Verification items for the finished model (mm, model axes). A direction names the side the tool comes from. Give positions to 0.01 mm unless a question says otherwise; leave off trailing zeros. Write each loop counter-clockwise with the first axis right and the second up, starting at its lowest first coordinate (ties: lowest second). Pieces come first, ordered by that corner, then holes. Notation, with made-up numbers: (-28.5, 42.5) -> (-19.5, 42.5) arc R22 cw to (-19.5, 76.5) -> close; hole circle Ø11 at (25.25, 76.25). An arc over 180 degrees is marked (long way). Answer as CSV lines item,"result".
```python
from build123d import *

# Parameters (mm, degrees)
F0_W     = 120
F0_H     = 118
F1_DEPTH = 4
F2_W     = 1
F2_H     = 1
F2_W_2   = 113
F2_H_2   = 111
F3_DEPTH = 2.5
F4_W     = 113
F4_H     = 111
F5_DEPTH = 5
F6_R     = 4


with BuildPart() as f1:
    # F0 (on Top) → F1 (new body)
    with BuildSketch(Plane.XY):
        Rectangle(F0_W, F0_H)
    extrude(amount=F1_DEPTH)

    # F2 (on face) → F3 (join)
    with BuildSketch(Plane.XY.offset(4)):
        with Locations((-57, 56)):
            Rectangle(F2_W, F2_H)
        with Locations((0, 56)):
            Rectangle(F2_W_2, F2_H)
        with Locations((-57, 0)):
            Rectangle(F2_W, F2_H_2)
        with Locations((57, 56)):
            Rectangle(F2_W, F2_H)
        with Locations((-57, -56)):
            Rectangle(F2_W, F2_H)
        with Locations((0, -56)):
            Rectangle(F2_W_2, F2_H)
        with Locations((57, 0)):
            Rectangle(F2_W, F2_H_2)
        with Locations((57, -56)):
            Rectangle(F2_W, F2_H)
    extrude(amount=F3_DEPTH)

    # F4 (on face) → F5 (cut)
    with BuildSketch(Plane.XY.offset(4)):
        Rectangle(F4_W, F4_H)
    extrude(amount=-F5_DEPTH, mode=Mode.SUBTRACT)

    # F6
    f6_edges = [f1.edges().sort_by_distance(p)[0] for p in [
        (-60, 59, 2),
        (60, 59, 2),
        (60, -59, 2),
        (-60, -59, 2),
    ]]
    fillet(f6_edges, radius=F6_R)


solid = f1.part
```
1) Section check C-C (z = 1.5). Record the boundary of the cut face in (x, y), and give its area (3 significant figures).
Reported:
outline,"(-60, -55) arc R4 ccw to (-56, -59) -> (56, -59) arc R4 ccw to (60, -55) -> (60, 55) arc R4 ccw to (56, 59) -> (-56, 59) arc R4 ccw to (-60, 55) -> close; hole (-56.5, -55.5) -> (56.5, -55.5) -> (56.5, 55.5) -> (-56.5, 55.5) -> close"
area,"1,600 mm²"
2) Tool access check on faces 1 (the flat face through (56.5, -1, 3)), 2 (the flat face through (60, -1, 2)). Record the directions out of +Z, -Z, +X, -X, +Y, -Y that give a thin tool (end or side, any length) a straight path to the whole face; none if there is none.
Reported:
face 1,"+Z, -Z"
face 2,"+Z, -Z, +X, +Y, -Y"
3) Draft check along Y on faces 3 (the flat face through (-1, 55.5, 3)), 4 (the flat face through (-5, -57, 0)), 5 (the flat face through (-1, 59, 2)). Enter one of: +Y half, -Y half, draft (parallel to the pull), parting line (faces both ways), or undercut.
Reported:
face 3,"undercut"
face 4,"draft"
face 5,"+Y half"
4) Scan lines: line 1 along Y through (x, z) = (14.5, 2.5); line 2 along X through (y, z) = (30, 2); line 3 along Y through (x, z) = (37.5, 5.75). Record each from-to range of solid material in increasing order.
Reported:
line 1,"-59 to -55.5, 55.5 to 59"
line 2,"-60 to -56.5, 56.5 to 60"
line 3,"-56.5 to -55.5, 55.5 to 56.5"
5) Depth check by flat-ended pin: pin 1 (0.8 mm diameter, centred on y = 11.5, z = 4.5, fed in from +X); pin 2 (0.8 mm diameter, centred on x = 19.5, z = 4.5, fed in from -Y); pin 3 (1.2 mm diameter, centred on x = -5, z = 5.5, fed in from +Y). Enter the tip coordinate at first touch or a pass-through.
Reported:
pin 1,"x = 57.5"
pin 2,"y = -56.5"
pin 3,"y = 56.5"
6) Section check B-B (x = 19). Record the boundary of the cut face in (y, z).
Reported:
outline,"(-59, 0) -> (-55.5, 0) -> (-55.5, 6.5) -> (-56.5, 6.5) -> (-56.5, 4) -> (-59, 4) -> close; (55.5, 0) -> (59, 0) -> (59, 4) -> (56.5, 4) -> (56.5, 6.5) -> (55.5, 6.5) -> close"
7) Section check A-A (y = 6.5). Record the boundary of the cut face in (x, z), and give its area (3 significant figures).
Reported:
outline,"(-60, 0) -> (-56.5, 0) -> (-56.5, 6.5) -> (-57.5, 6.5) -> (-57.5, 4) -> (-60, 4) -> close; (56.5, 0) -> (60, 0) -> (60, 4) -> (57.5, 4) -> (57.5, 6.5) -> (56.5, 6.5) -> close"
area,"33.0 mm²"
